from build123d import *

# Parameters (mm, degrees)
SKIZZE1_W                  = 350
SKIZZE1_H                  = 250
GRUNDPLATTE_DEPTH          = 5
SKIZZE2_W                  = 38
SKIZZE2_H                  = 5
ZAPFEN_BODEN_DEPTH         = 6
SKIZZE3_R                  = 5
VERBINDUNGSBOHRUNGEN_DEPTH = 6


with BuildPart() as part:
    # Skizze1 → Grundplatte (new body)
    with BuildSketch(Plane(origin=(0, 0, 0), x_dir=(0, 0, -1), z_dir=(1, 0, 0))):
        with Locations((0, 125)):
            Rectangle(SKIZZE1_W, SKIZZE1_H)
    extrude(amount=GRUNDPLATTE_DEPTH)

    # Skizze2 → Zapfen Boden (cut, through all)
    with BuildSketch(Plane(origin=(5, 0, 0), x_dir=(0, 0, -1), z_dir=(1, 0, 0))):
        with Locations((-156, 2.5)):
            Rectangle(SKIZZE2_W, SKIZZE2_H)
        with Locations((-78, 2.5)):
            Rectangle(SKIZZE2_W, SKIZZE2_H)
        with Locations((0, 2.5)):
            Rectangle(SKIZZE2_W, SKIZZE2_H)
        with Locations((78, 2.5)):
            Rectangle(SKIZZE2_W, SKIZZE2_H)
        with Locations((156, 2.5)):
            Rectangle(SKIZZE2_W, SKIZZE2_H)
    extrude(amount=-ZAPFEN_BODEN_DEPTH, mode=Mode.SUBTRACT)

    # Skizze3 → Verbindungsbohrungen (cut, through all)
    with BuildSketch(Plane(origin=(5, 0, 0), x_dir=(0, 0, -1), z_dir=(1, 0, 0))):
        with Locations((145, 220)):
            Circle(SKIZZE3_R)
        with Locations((-145, 220)):
            Circle(SKIZZE3_R)
        with Locations((-145, 35)):
            Circle(SKIZZE3_R)
        with Locations((145, 35)):
            Circle(SKIZZE3_R)
    extrude(amount=-VERBINDUNGSBOHRUNGEN_DEPTH, mode=Mode.SUBTRACT)


solid = part.part
Can you work these out from the model? Positions are in its coordinate system, mm. Coordinates: 2 decimals unless noted, no trailing zeros. Write each loop counter-clockwise with the first axis right and the second up, starting at its lowest first coordinate (ties: lowest second). Pieces come first, ordered by that corner, then holes. Notation, with made-up numbers: (45, -1.75) -> (100, -1.75) arc R8 cw to (100, 13.25) -> close; hole circle Ø9 at (12.5, 38.5). An arc over 180 degrees is marked (long way). Write each question's results on one line, items separated by ' | '. Start each with the question number.
Q1. Imagine slicing it at B-B (z = 145). Write out the boundary of the cut face in (x, y).
Q2. I'm going to push flat-ended pins straight in: pin 1 (2.5 mm diameter, centred on x = 1.5, y = 2, fed in from +Z); pin 2 (2.5 mm diameter, centred on x = 3.5, y = 2, fed in from -Z); pin 3 (1.5 mm diameter, centred on x = 1.5, z = -9, fed in from -Y); pin 4 (6 mm diameter, centred on y = 220, z = 145, fed in from -X). Where does each tip first touch, or does it pass through?
Q3. If I drill on probe 1 along Y at (x, z) = (3.8, 145); probe 2 along Y at (x, z) = (1.1, -90), over which ranges is the centre line in solid material (lowest first)?
Q4. Imagine slicing it at A-A (y = 220). Write out the boundary of the cut face in (x, z).
Q5. Imagine slicing it at C-C (z = -1.5). Write out the boundary of the cut face in (x, y).
Q6. We'd pull the mould along Z, two halves only. Please class faces 1 (the face through (5, 127, 2)), 2 (the face through (2.535, 224.957, -144.349)): +Z half, -Z half, draft (parallel to the pull), parting line (faces both ways), or undercut.
Taken from the geometry:
1) outline: (0, 5) -> (5, 5) -> (5, 30) -> (0, 30) -> close; (0, 40) -> (5, 40) -> (5, 215) -> (0, 215) -> close; (0, 225) -> (5, 225) -> (5, 250) -> (0, 250) -> close
2) pin 1: stops at z = 137 | pin 2: stops at z = -137 | pin 3: stops at y = 5 | pin 4: passes through
3) probe 1: y = 5 to 30, 40 to 215, 225 to 250 | probe 2: y = 5 to 250
4) outline: (0, -175) -> (5, -175) -> (5, -150) -> (0, -150) -> close; (0, -140) -> (5, -140) -> (5, 140) -> (0, 140) -> close; (0, 150) -> (5, 150) -> (5, 175) -> (0, 175) -> close
5) outline: (0, 5) -> (5, 5) -> (5, 250) -> (0, 250) -> close
6) face 1: draft | face 2: undercut
